Here's how the part is built. I have some questions about the finished solid (model axes, mm). A direction names the side the tool comes from. Coordinates: 2 decimals unless noted, no trailing zeros. Write each loop counter-clockwise with the first axis right and the second up, starting at its lowest first coordinate (ties: lowest second). Pieces come first, ordered by that corner, then holes.
```python
from build123d import *

# Parameters (mm, degrees)
SKETCH_1_W          = 30
SKETCH_1_H          = 30
SKETCH_1_W_2        = 27.6
SKETCH_1_H_2        = 27.6
EXTRUDE_1_DEPTH     = 295
SKETCH_2_R          = 2
CUT_EXTRUDE_1_DEPTH = 10
SKETCH_3_R          = 4
CUT_EXTRUDE_2_DEPTH = 10
CUT_EXTRUDE_3_DEPTH = 111
SKETCH_5_R          = 2
CUT_EXTRUDE_4_DEPTH = 10
SKETCH_6_R          = 2
CUT_EXTRUDE_5_DEPTH = 10
SKETCH_7_R          = 1.5
CUT_EXTRUDE_6_DEPTH = 10
SKETCH_8_R          = 2
CUT_EXTRUDE_7_DEPTH = 46
SKETCH_9_R          = 4
CUT_EXTRUDE_8_DEPTH = 5


with BuildPart() as part:
    # 草图1 → 凸台-拉伸1 (new, symmetric)
    with BuildSketch(Plane.XY):
        Rectangle(SKETCH_1_W, SKETCH_1_H)
        Rectangle(SKETCH_1_W_2, SKETCH_1_H_2, mode=Mode.SUBTRACT)
    extrude(amount=EXTRUDE_1_DEPTH, both=True)

    # 草图2 → 切除-拉伸1 (cut)
    with BuildSketch(Plane(origin=(0, 15, 0), x_dir=(1, 0, 0), z_dir=(0, 1, 0))):
        with Locations(Location((-9, 220, 0), (0, 0, 270))):
            Circle(SKETCH_2_R)
        with Locations(Location((9, 220, 0), (0, 0, 270))):
            Circle(SKETCH_2_R)
        with Locations(Location((-9, 240, 0), (0, 0, 270))):
            Circle(SKETCH_2_R)
        with Locations(Location((9, 240, 0), (0, 0, 270))):
            Circle(SKETCH_2_R)
        with Locations((9, -240)):
            Circle(SKETCH_2_R)
        with Locations((-9, -240)):
            Circle(SKETCH_2_R)
        with Locations((9, -220)):
            Circle(SKETCH_2_R)
        with Locations((-9, -220)):
            Circle(SKETCH_2_R)
    extrude(amount=-CUT_EXTRUDE_1_DEPTH, mode=Mode.SUBTRACT)

    # 草图3 → 切除-拉伸2 (cut)
    with BuildSketch(Plane(origin=(0, -13.8, 0), x_dir=(1, 0, 0), z_dir=(0, 1, 0))):
        with Locations(Location((-9, 240, 0), (0, 0, 270))):
            Circle(SKETCH_3_R)
        with Locations(Location((9, 240, 0), (0, 0, 270))):
            Circle(SKETCH_3_R)
        with Locations(Location((-9, 220, 0), (0, 0, 270))):
            Circle(SKETCH_3_R)
        with Locations(Location((9, 220, 0), (0, 0, 270))):
            Circle(SKETCH_3_R)
        with Locations(Location((9, -220, 0), (0, 0, 270))):
            Circle(SKETCH_3_R)
        with Locations(Location((-9, -220, 0), (0, 0, 270))):
            Circle(SKETCH_3_R)
        with Locations(Location((9, -240, 0), (0, 0, 270))):
            Circle(SKETCH_3_R)
        with Locations(Location((-9, -240, 0), (0, 0, 270))):
            Circle(SKETCH_3_R)
    extrude(amount=-CUT_EXTRUDE_2_DEPTH, mode=Mode.SUBTRACT)

    # 草图4 → 切除-拉伸3 (cut)
    with BuildSketch(Plane(origin=(15, 0, 0), x_dir=(0, 0, -1), z_dir=(1, 0, 0))):
        with BuildLine():
            Line((-135, 8), (-125, 8))
            ThreePointArc((-125, 8), (-117, 0), (-125, -8))
            Line((-125, -8), (-135, -8))
            ThreePointArc((-135, -8), (-143, 0), (-135, 8))
        make_face()
    cut_extrude_3 = extrude(amount=-CUT_EXTRUDE_3_DEPTH, mode=Mode.SUBTRACT)

    # 镜向1: 切除-拉伸3 across plane
    add(cut_extrude_3.mirror(Plane.XY), mode=Mode.SUBTRACT)

    # 草图5 → 切除-拉伸4 (cut)
    with BuildSketch(Plane(origin=(0, 15, 0), x_dir=(1, 0, 0), z_dir=(0, 1, 0))):
        with Locations(Location((-9, -139, 0), (0, 0, 270))):
            Circle(SKETCH_5_R)
        with Locations(Location((-9, -121, 0), (0, 0, 270))):
            Circle(SKETCH_5_R)
        with Locations(Location((9, -121, 0), (0, 0, 270))):
            Circle(SKETCH_5_R)
        with Locations(Location((9, -139, 0), (0, 0, 270))):
            Circle(SKETCH_5_R)
    cut_extrude_4 = extrude(amount=-CUT_EXTRUDE_4_DEPTH, mode=Mode.SUBTRACT)

    # 镜向2: 切除-拉伸4 across plane
    add(cut_extrude_4.mirror(Plane.XY), mode=Mode.SUBTRACT)

    # 草图6 → 切除-拉伸5 (cut)
    with BuildSketch(Plane(origin=(0, 15, 0), x_dir=(1, 0, 0), z_dir=(0, 1, 0))):
        with Locations(Location((-9, -285, 0), (0, 0, 270))):
            Circle(SKETCH_6_R)
        with Locations(Location((9, -285, 0), (0, 0, 270))):
            Circle(SKETCH_6_R)
    cut_extrude_5 = extrude(amount=-CUT_EXTRUDE_5_DEPTH, mode=Mode.SUBTRACT)

    # 镜向3: 切除-拉伸5 across plane
    add(cut_extrude_5.mirror(Plane.XY), mode=Mode.SUBTRACT)

    # 草图7 → 切除-拉伸6 (cut)
    with BuildSketch(Plane.XZ.offset(15)):
        with Locations(Location((0, 98.738437042, 0), (0, 0, 270))):
            Circle(SKETCH_7_R)
        with Locations(Location((0, 38.738437042, 0), (0, 0, 270))):
            Circle(SKETCH_7_R)
        with Locations(Location((0, -38.738437042, 0), (0, 0, 270))):
            Circle(SKETCH_7_R)
        with Locations(Location((0, -98.738437042, 0), (0, 0, 270))):
            Circle(SKETCH_7_R)
    extrude(amount=-CUT_EXTRUDE_6_DEPTH, mode=Mode.SUBTRACT)

    # 草图8 → 切除-拉伸7 (cut, symmetric)
    with BuildSketch(Plane.XZ.offset(-13.8)):
        with Locations((8.95, 206.45)):
            Circle(SKETCH_8_R)
        with Locations((-8.95, 206.45)):
            Circle(SKETCH_8_R)
        with Locations((-8.95, 188.55)):
            Circle(SKETCH_8_R)
        with Locations((8.95, 188.55)):
            Circle(SKETCH_8_R)
    cut_extrude_7 = extrude(amount=CUT_EXTRUDE_7_DEPTH, both=True, mode=Mode.SUBTRACT)

    # 镜向4: 切除-拉伸7 across plane
    add(cut_extrude_7.mirror(Plane.XY), mode=Mode.SUBTRACT)

    # 草图9 → 切除-拉伸8 (cut, symmetric)
    with BuildSketch(Plane.XZ.offset(15)):
        with Locations(Location((-8.95, 206.45, 0), (0, 0, 90))):
            Circle(SKETCH_9_R)
        with Locations(Location((8.95, 206.45, 0), (0, 0, 90))):
            Circle(SKETCH_9_R)
        with Locations(Location((8.95, 188.55, 0), (0, 0, 90))):
            Circle(SKETCH_9_R)
        with Locations(Location((-8.95, 188.55, 0), (0, 0, 90))):
            Circle(SKETCH_9_R)
        with Locations(Location((-8.95, -188.55, 0), (0, 0, 90))):
            Circle(SKETCH_9_R)
        with Locations(Location((8.95, -188.55, 0), (0, 0, 90))):
            Circle(SKETCH_9_R)
        with Locations(Location((8.95, -206.45, 0), (0, 0, 90))):
            Circle(SKETCH_9_R)
        with Locations(Location((-8.95, -206.45, 0), (0, 0, 90))):
            Circle(SKETCH_9_R)
    extrude(amount=CUT_EXTRUDE_8_DEPTH, both=True, mode=Mode.SUBTRACT)


solid = part.part
```
1) We'd pull the mould along X, two halves only. Please class faces 3 (the face through (-15, 0, 4)), 4 (the face through (0, -15, 4)), 5 (the face through (0, 13.8, 4)): pulls with the +X half, pulls with the -X half, needs draft (parallel to the pull), parting line crosses it, or undercut.
Values follow:
face 3: pulls with the -X half
face 4: needs draft
face 5: undercut
2) Imagine slicing it at B-B on z = 251.5. Please give me the cut outline in (x, y), then the cut area to 3 significant figures.
Values follow:
outline: (-15, -15) - (15, -15) - (15, 15) - (-15, 15) - close; hole (-13.8, -13.8) - (13.8, -13.8) - (13.8, 13.8) - (-13.8, 13.8) - close
area: 138 mm2
3) On a 3-axis mill with a long thin cutter (end or side, diameter ignored), from which of +Z, -Z, +X, -X, +Y, -Y can I reach the whole of each face in a straight line? I mean faces 1 (the face through (13.8, 0, 4)), 2 (the face through (0, 15, 4)). Say none if no direction works.
Values follow:
face 1: +Z, -Z
face 2: +Z, -Z, +X, -X, +Y
4) Will this pin go through, and if not, where does the flat tip stop? pin 1 (4.5 mm diameter, centred on x = 8.95, z = 188.55, fed in from +Y).
Values follow:
pin 1: stops at y = 15
5) Imagine slicing it at A-A on y = 0. Please give me the cut outline in (x, z), then the cut area to 3 significant figures.
Values follow:
outline: (-15, -295) - (-13.8, -295) - (-13.8, -143) - (-15, -143) - close; (-15, -117) - (-13.8, -117) - (-13.8, 117) - (-15, 117) - close; (-15, 143) - (-13.8, 143) - (-13.8, 295) - (-15, 295) - close; (13.8, -295) - (15, -295) - (15, -143) - (13.8, -143) - close; (13.8, -117) - (15, -117) - (15, 117) - (13.8, 117) - close; (13.8, 143) - (15, 143) - (15, 295) - (13.8, 295) - close
area: 1,290 mm2
6) I need wall thicknesses on probe 1 along X at (y, z) = (-14.6, 206.45); probe 2 along X at (y, z) = (-5.5, 207.5). Which ranges of each line are inside material? Lowest first, please.
Values follow:
probe 1: x = -15 to -12.95, -4.95 to 4.95, 12.95 to 15
probe 2: x = -15 to -13.8, 13.8 to 15
